Input: part model. Units: mm. Frame: model coordinates. Face numbers are marked on the shaded views. A direction names the side the tool comes from. Coordinates: 2 decimals unless noted, no trailing zeros. Write each loop counter-clockwise with the first axis right and the second up, starting at its lowest first coordinate (ties: lowest second). Pieces come first, ordered by that corner, then holes. Notation, with made-up numbers: (-26.75, 60.25) -> (11.25, 60.25) arc R16 ccw to (11.25, 74.25) -> close; hole circle Ø7 at (-28, -9.75). An arc over 180 degrees is marked (long way). One line per question, with ' | ' between items. Start each with the question number.
```python
from build123d import *

# Parameters (mm, degrees)
SKETCH_1_R          = 1.5
EXTRUDE_1_DEPTH     = 2
SKETCH_2_R          = 2.95
EXTRUDE_2_DEPTH     = 0.95
CUT_EXTRUDE_1_DEPTH = 1
SKETCH_1_8_R        = 1.5
EXTRUDE_5_DEPTH     = 5


with BuildPart() as part:
    # Sketch 1 → Extrude 1 (new body)
    with BuildSketch(Plane(origin=(0, 0, 0), x_dir=(1, 0, 0), z_dir=(0, 1, 0))):
        with Locations(Location((0, 0, 0), (0, 0, 270))):
            Circle(SKETCH_1_R)
    extrude(amount=EXTRUDE_1_DEPTH)

    # Sketch 2 → Extrude 2 (add)
    with BuildSketch(Plane(origin=(0, 0, 0), x_dir=(-1, 0, 0), z_dir=(0, 1, 0))):
        with Locations(Location((0, 0, 0), (0, 0, 90))):
            Circle(SKETCH_2_R)
    extrude(amount=-EXTRUDE_2_DEPTH)

    # Sketch 4 → Cut-Revolve 1 (revolve, cut)
    with BuildSketch(Plane(origin=(0, 0, 0), x_dir=(0, 0, -1), z_dir=(1, 0, 0))):
        with BuildLine():
            Line((-2.901374674, 0), (-2.95, 0))
            Line((-2.95, 0), (-2.95, -0.95))
            Line((-2.95, -0.95), (-2.901374674, -0.95))
            ThreePointArc((-2.901374674, -0.95), (-2.94, -0.475), (-2.901374674, 0))
        make_face()
    revolve(axis=Axis((0, 3.165730861, 0), (0, -1, 0)), mode=Mode.SUBTRACT)

    # Sketch 3 → Cut-Extrude 1 (cut)
    with BuildSketch(Plane.XZ.offset(0.95)):
        Polygon((-1.177794549, 0), (-0.588897275, -1.02), (0.588897275, -1.02), (1.177794549, 0), (0.588897275, 1.02), (-0.588897275, 1.02), align=None)
    extrude(amount=-CUT_EXTRUDE_1_DEPTH, mode=Mode.SUBTRACT)

    # Sketch 1_8 → Extrude 5 (add)
    with BuildSketch(Plane(origin=(0, 0, 0), x_dir=(1, 0, 0), z_dir=(0, 1, 0))):
        with Locations(Location((0, 0, 0), (0, 0, 270))):
            Circle(SKETCH_1_8_R)
    extrude(amount=EXTRUDE_5_DEPTH)


solid = part.part
```
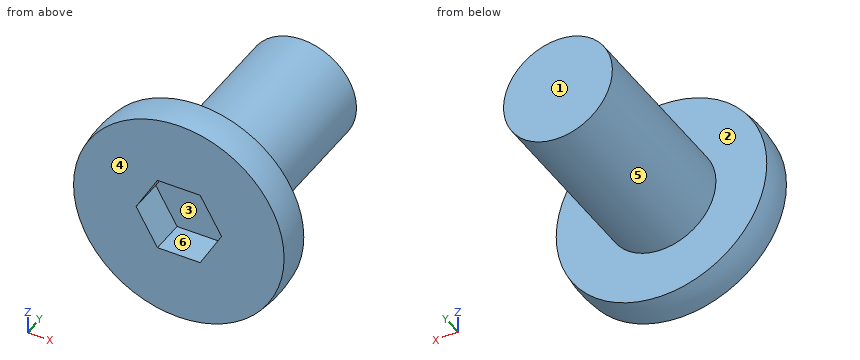
1) Pull-direction query (Z, two-part tool) for the marked faces 4, 5 and 6; classes: released by +Z, released by -Z, zero draft, split by the parting line, or undercut.
2) Section C-C, the plane y = 0.65. Return loops of the section in (x, z), then the cut area to 3 significant figures.
3) Section A-A, the plane x = 0. Return loops of the section in (y, z) (3 decimals).
4) Ray query, line 1 (Y direction, x = 1.65, z = 1); line 2 (X direction, y = 0.55, z = 0.05); line 3 (Y direction, x = 0.5, z = -0.85). Return the intervals inside material, ascending.
5) First-contact query: P1, Ø2, axis at x = -2, z = -2.5, coming from the +Y side; P2, Ø3, axis at x = 1.5, z = -2.5, coming from the +Y side; P3, Ø1, axis at x = 0.5, z = 0, coming from the -Y side. Flat tips, straight axial feed; report the tip coordinate or a pass-through.
6) Section D-D, the plane z = 1.9. Return loops of the section in (x, y) (3 decimals), then the cut area to 3 significant figures.
7) Section B-B, the plane z = -0.7. Return loops of the section in (x, y) (3 decimals).
8) Access query for the marked faces 1, 2 and 3. Directions: +Z, -Z, +X, -X, +Y, -Y. A direction counts if a zero-diameter tool reaches every point of the face in a straight line with its end or side. Return the directions, or none.
Answer block:
1) face 4: zero draft | face 5: split by the parting line | face 6: undercut
2) outline: circle Ø3 at (0, 0) | area: 7.07 mm2
3) outline: (-0.95, -2.901) arc R2.94 ccw to (0, -2.901) -> (0, -1.5) -> (5, -1.5) -> (5, 1.5) -> (0, 1.5) -> (0, 2.901) arc R2.94 ccw to (-0.95, 2.901) -> (-0.95, 1.02) -> (0, 1.02) -> (0, -1.02) -> (-0.95, -1.02) -> close
4) line 1: y = -0.95 to 0 | line 2: x = -1.5 to 1.5 | line 3: y = 0 to 5
5) P1: stops at y = 0 | P2: stops at y = 5 | P3: stops at y = 0
6) outline: (-2.193, -0.95) -> (2.193, -0.95) arc R2.244 ccw to (2.193, 0) -> (-2.193, 0) arc R2.244 ccw to start | area: 4.23 mm2
7) outline: (-2.816, -0.95) -> (-0.774, -0.95) -> (-0.774, 0) -> (0.774, 0) -> (0.774, -0.95) -> (2.816, -0.95) arc R2.855 ccw to (2.816, 0) -> (1.327, 0) -> (1.327, 5) -> (-1.327, 5) -> (-1.327, 0) -> (-2.816, 0) arc R2.855 ccw to start
8) face 1: +Z, -Z, +X, -X, +Y | face 2: +Y | face 3: -Y
